Work out the finished part from the listing and answer in its coordinate system (mm). A direction names the side the tool comes from. Give positions to 0.01 mm unless a question says otherwise; leave off trailing zeros. Write each loop counter-clockwise with the first axis right and the second up, starting at its lowest first coordinate (ties: lowest second). Pieces come first, ordered by that corner, then holes. Notation, with made-up numbers: (-38.5, 35.25) -> (-31.5, 35.25) arc R6 cw to (-31.5, 46.25) -> close; hole circle Ø6 at (43, -7.75). An arc over 180 degrees is marked (long way). Use a Markdown table: item, result. Add a question column.
Q1. For faces 1 (the face through (-18.538, 4.885, -4.93)), 2 (the face through (-16.07, -30.18, -4.93)), 3 (the face through (-8, -14, -6)), 4 (the face through (43.91, -7.52, -4.93)), determine the directions among +Z, -Z, +X, -X, +Y, -Y from which every point of the face is accessible in a straight line to the end or side of a thin tool.
Q2. For a pull along Y with two mould halves and no side action, classify faces 5 (the face through (-18.003, 2.676, -8.028)), 6 (the face through (-89, -74.153, -4)), 7 (the face through (35.51, 23.69, -4.93)), 8 (the face through (-10, 1, -10)) as pulls with the +Y half, pulls with the -Y half, needs draft (parallel to the pull), parting line crosses it, or undercut.
Q3. Section D-D, the plane y = -21.5 is taken. Give the vertices of the cut face in (x, z), plus the area to 3 significant figures.
Q4. Each of these flat-tipped pins is pushed along its axis until it touches: pin 1 Ø6 at (x, z) = (-60.5, -8.5) entering from -Y; pin 2 Ø2 at (y, z) = (34, -3) entering from -X; pin 3 Ø5 at (x, y) = (-85.5, -58.5) entering from -Z; pin 4 Ø6 at (x, y) = (-71.49, -55.1) entering from -Z. Where does it stop, or does it pass through?
Q5. Section B-B, the plane z = -4 is taken. Give the vertices of the cut face in (x, y), plus the area to 3 significant figures.
Q6. Section C-C, the plane x = -26 is taken. Give the vertices of the cut face in (y, z).
Q7. Consider line 1 (Z direction, x = -1.5, y = -10); line 2 (Y direction, x = 18.5, z = -8.5); line 3 (Y direction, x = -13.5, z = -6.5). Determine where each line is inside the solid, lowest interval first.
Q8. Section A-A, the plane y = -52.5 is taken. Give the vertices of the cut face in (x, z), plus the area to 3 significant figures.
from build123d import *

# Parameters (mm, degrees)
SKETCH1_R           = 5
BOSS_EXTRUDE1_DEPTH = 10
CUT_EXTRUDE1_DEPTH  = 4


with BuildPart() as part:
    # Sketch1 → Boss-Extrude1 (new body)
    with BuildSketch(Plane.XY):
        Polygon((72.027126309, 48.055346158), (89.027642078, 17.992338813), (-2.487468662, -33.759106586), (-30.037099765, -26.499406498), (-70.803107952, -74.152822461), (-108.242490343, -74.152822461), (-36.564435859, 9.635222963), (0, 0), align=None)
        with Locations((-71.49077455, -55.104728104)):
            Circle(SKETCH1_R, mode=Mode.SUBTRACT)
    extrude(amount=-BOSS_EXTRUDE1_DEPTH)

    # Sketch2 → Cut-Extrude1 (cut)
    with BuildSketch(Plane(origin=(0, 0, -10), x_dir=(-1, 0, 0), z_dir=(0, 0, -1))):
        Polygon((-71.346056645, 45.196672444), (-73.014288261, 46.309689884), (-88.043159753, 19.733256545), (-86.30224202, 18.74877422), (2.764141771, -31.617925447), (30.741045074, -24.245633361), (71.72414825, -72.152822461), (73.43508575, -74.152822461), (105.610512545, -74.152822461), (103.899575045, -72.152822461), (35.86049055, 7.381449825), (-0.361020517, -2.163407821), align=None)
    extrude(amount=-CUT_EXTRUDE1_DEPTH, mode=Mode.SUBTRACT)


solid = part.part
Result set:
| question | item | result |
|---|---|---|
| 1 | face 1 | +Z, -Z, +Y |
| 1 | face 2 | +Z, -Z, -Y |
| 1 | face 3 | -Z |
| 1 | face 4 | +Z, -Z, +X, -Y |
| 2 | face 5 | undercut |
| 2 | face 6 | pulls with the -Y half |
| 2 | face 7 | pulls with the +Y half |
| 2 | face 8 | needs draft |
| 3 | outline | (-63.2, -10) -> (-60.57, -10) -> (-60.57, -6) -> (15.13, -6) -> (15.13, -10) -> (19.19, -10) -> (19.19, 0) -> (-63.2, 0) -> close |
| 3 | area | 521 mm2 |
| 4 | pin 1 | stops at y = -65.62 |
| 4 | pin 2 | stops at x = 49.46 |
| 4 | pin 3 | stops at z = -6 |
| 4 | pin 4 | passes through |
| 5 | outline | (-108.24, -74.15) -> (-70.8, -74.15) -> (-30.04, -26.5) -> (-2.49, -33.76) -> (89.03, 17.99) -> (72.03, 48.06) -> (0, 0) -> (-36.56, 9.64) -> close; hole circle Ø10 at (-71.49, -55.1) |
| 5 | area | 6,460 mm2 |
| 6 | outline | (-27.56, -10) -> (-25.49, -10) -> (-25.49, -6) -> (4.78, -6) -> (4.78, -10) -> (6.85, -10) -> (6.85, 0) -> (-27.56, 0) -> close |
| 7 | line 1 | z = -6 to 0 |
| 7 | line 2 | y = -21.89 to -19.59, 9.94 to 12.34 |
| 7 | line 3 | y = -30.86 to -28.79, 1.49 to 3.56 |
| 8 | outline | (-89.72, -10) -> (-87.09, -10) -> (-87.09, -6) -> (-75.76, -6) -> (-75.76, 0) -> (-89.72, 0) -> close; (-67.22, -6) -> (-54.91, -6) -> (-54.91, -10) -> (-52.28, -10) -> (-52.28, 0) -> (-67.22, 0) -> close |
| 8 | area | 194 mm2 |
